Source: CAD feature listing. Evaluate the final solid. Frame: model axes, mm. Face numbers are marked on the shaded views. A direction names the side the tool comes from. Round coordinates to 2 decimals unless told otherwise and drop trailing zeros. Order: outer loops, then holes, each group sorted by start corner. A loop starts at its lowest first (then second) coordinate and runs counter-clockwise, first axis right, second up. Notation, with made-up numbers: (21.25, 87) -> (26.25, 87) arc R18 ccw to (26.25, 119) -> close; hole circle Ø7 at (18, 75). An arc over 180 degrees is marked (long way). One line per item, written item: value. Start each with the question number.
1) Section B-B (y = 1). Return the cut outline in (x, z), and give its area (3 significant figures).
2) Section C-C (x = 1). Return the cut outline in (y, z).
3) Ray query, L1, parallel to X at y = 0.25, z = 1.25; L2, parallel to X at y = 2, z = 1.6; L3, parallel to Y at x = 3.75, z = 2.7. Return the intervals inside material, ascending.
4) Reachability of the marked faces 4, 5, 6 and 7 from +Z, -Z, +X, -X, +Y, -Y: full face, straight path, thin tool, end or side. Return the list, or none.
5) Section A-A (x = -3.5). Return the cut outline in (y, z), and give its area (3 significant figures).
6) Pin query (flat end, axial travel): P1, Ø1, axis at y = 2.5, z = 2.5, coming from the +X side (3 decimals); P2, Ø0.9, axis at x = -4, z = 2, coming from the +Y side; P3, Ø0.9, axis at y = -5.5, z = 1.5, coming from the -X side. Return the tip coordinate at first contact, or that it passes through.
7) Section D-D (y = -3.5). Return the cut outline in (x, z), and give its area (3 significant figures).
8) Mould query, pull axis Y, two halves, no side actions, for the marked faces 1, 2 and 3. Classes: pulls with the +Y half, pulls with the -Y half, needs draft (parallel to the pull), parting line crosses it, or undercut.
```python
from build123d import *

# Parameters (mm, degrees)
F2_DEPTH = 3
F4_DEPTH = 2.6
F5_R     = 0.49999
F6_R     = 1.4


# Not quite as in the source:
# - a fillet or chamfer is up to 0.001 mm smaller than in the source, because OpenCascade refuses the exact size


with BuildPart() as f2:
    # F1 (on Top) → F2 (new body)
    with BuildSketch(Plane.XY):
        Polygon((2.8, 1.4), (2.8, 4), (-2.8, 4), (-2.8, 1.4), (-1.5, 1.4), (-1.5, 0), (-4.5, 0), (-4.5, 0.5), (-5.6, 0.5), (-6.1, 0), (-7.5, 0), (-7.5, -3.0118150752), (-1.4735722734, -3.0118150752), (-1.4735722734, -4.5618148234), (-5.01158851, -4.5618148234), (-5.01158851, -6.3443139292), (5.01158851, -6.3443139292), (5.01158851, -4.5618148234), (1.4735722734, -4.5618148234), (1.4735722734, -3.0118150752), (7.5, -3.0118150752), (7.5, 0), (6.1, 0), (5.6, 0.5), (4.5, 0.5), (4.5, 0), (1.5, 0), (1.5, 1.4), align=None)
    extrude(amount=F2_DEPTH)

    # F3 (on face) → F4 (cut, through all)
    with BuildSketch(Plane(origin=(0, 4, 0), x_dir=(-1, 0, 0), z_dir=(0, 1, 0))):
        with BuildLine():
            Line((2.8, 0), (2.8, 1.5))
            ThreePointArc((2.8, 1.5), (2.6888743587, 0.7190040441), (2.3643180835, 0))
            Line((2.3643180835, 0), (2.8, 0))
        make_face()
        with BuildLine():
            ThreePointArc((2.3643180835, 3), (2.6888743587, 2.2809959559), (2.8, 1.5))
            Line((2.8, 1.5), (2.8, 3))
            Line((2.8, 3), (2.3643180835, 3))
        make_face()
        with BuildLine():
            ThreePointArc((-2.3643180835, 0), (0, -1.3), (2.3643180835, 0))
            Line((2.3643180835, 0), (-2.3643180835, 0))
        make_face()
        with BuildLine():
            ThreePointArc((-2.8, 1.5), (-2.6888743587, 2.2809959559), (-2.3643180835, 3))
            Line((-2.3643180835, 3), (-2.8, 3))
            Line((-2.8, 3), (-2.8, 1.5))
        make_face()
        with BuildLine():
            Line((-2.8, 0), (-2.3643180835, 0))
            ThreePointArc((-2.3643180835, 0), (-2.6888743587, 0.7190040441), (-2.8, 1.5))
            Line((-2.8, 1.5), (-2.8, 0))
        make_face()
    extrude(amount=-F4_DEPTH, mode=Mode.SUBTRACT)

    # F5 (radius 0.5 in the source; OpenCascade refuses exactly that, so slightly less here)
    f5_edges = [f2.edges().sort_by_distance(p)[0] for p in [
        (4.5, 0.5, 1.5),
        (5.6, 0.5, 1.5),
        (7.5, 0, 1.5),
        (7.5, -3.011815, 1.5),
        (5.011589, -4.561815, 1.5),
        (5.011589, -6.344314, 1.5),
        (-4.5, 0.5, 1.5),
        (-5.6, 0.5, 1.5),
        (-7.5, 0, 1.5),
        (-7.5, -3.011815, 1.5),
        (-5.011589, -6.344314, 1.5),
        (-5.011589, -4.561815, 1.5),
        (2.364318, 2.7, 3),
        (-2.364318, 2.7, 3),
        (2.364318, 2.7, 0),
        (-2.364318, 2.7, 0),
    ]]
    fillet(f5_edges, radius=F5_R)

    # F6
    f6_edges = [f2.edges().sort_by_distance(p)[0] for p in [
        (1.5, 0.7, 3),
        (-1.5, 0.7, 3),
        (1.5, 0.7, 0),
        (-1.5, 0.7, 0),
    ]]
    fillet(f6_edges, radius=F6_R)


solid = f2.part
```
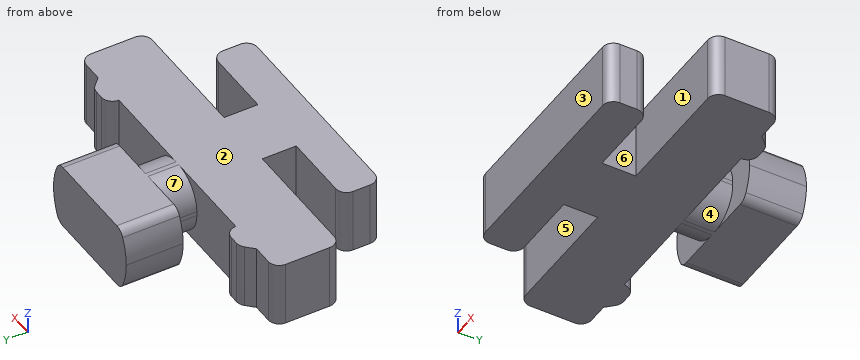
Findings:
1. outline: (-1.5, 1.4) arc R1.4 ccw to (-0.1, 0) -> (0.1, 0) arc R1.4 ccw to (1.5, 1.4) -> (1.5, 1.6) arc R1.4 ccw to (0.1, 3) -> (-0.1, 3) arc R1.4 ccw to (-1.5, 1.6) -> close
1. area: 7.32 mm2
2. outline: (-6.34, 0) -> (0, 0) -> (0, 0.33) -> (1.4, 0.33) -> (1.4, 0) -> (4, 0) -> (4, 3) -> (1.4, 3) -> (1.4, 2.67) -> (0, 2.67) -> (0, 3) -> (-6.34, 3) -> close
3. L1: -5.85 to -4.57, -1.49 to 1.49, 4.57 to 5.85
3. L2: -2.8 to 2.8
3. L3: -6.34 to -4.56, -3.01 to 0
4. face 4: -Z
4. face 5: +Z, -Z, -X
4. face 6: +Z, -Z, +X
4. face 7: +Z
5. outline: (-6.34, 0) -> (-4.56, 0) -> (-4.56, 3) -> (-6.34, 3) -> close; (-3.01, 0) -> (0, 0) -> (0, 3) -> (-3.01, 3) -> close
5. area: 14.4 mm2
6. P1: x = 2.755
6. P2: y = 0
6. P3: x = -5.01
7. outline: (-1.47, 0) -> (1.47, 0) -> (1.47, 3) -> (-1.47, 3) -> close
7. area: 8.84 mm2
8. face 1: undercut
8. face 2: needs draft
8. face 3: pulls with the -Y half
